from build123d import *

# Parameters (mm, degrees)
ESQUISSE1_R                                   = 3.9
BOSS_EXTRU_1_DEPTH                            = 105
ESQUISSE2_W                                   = 12
ESQUISSE2_H                                   = 12
BOSS_EXTRU_2_DEPTH                            = 5
ESQUISSE14_R                                  = 3.9
ESQUISSE14_R_2                                = 3
ENL_V_MAT_EXTRU_1_DEPTH                       = 6
CHANFREIN1_SIZE                               = 2
TROU_POUR_TARAUDAGE_POUR_TROU_TARAUD_M3_D     = 2.5
TROU_POUR_TARAUDAGE_POUR_TROU_TARAUD_M3_DEPTH = 12


with BuildPart() as part:
    # Esquisse1 → Boss.-Extru.1 (new body)
    with BuildSketch(Plane.XY):
        with Locations((-68.275651986, -15.580620135)):
            Circle(ESQUISSE1_R)
    extrude(amount=BOSS_EXTRU_1_DEPTH)

    # Esquisse2 → Boss.-Extru.2 (add)
    with BuildSketch(Plane.XY.offset(105)):
        with Locations((-68.275651986, -15.580620135)):
            Rectangle(ESQUISSE2_W, ESQUISSE2_H)
    extrude(amount=BOSS_EXTRU_2_DEPTH)

    # Esquisse14 → Enlèv. mat.-Extru.1 (cut)
    with BuildSketch(Plane(origin=(0, 0, 0), x_dir=(-1, 0, 0), z_dir=(0, 0, -1))):
        with Locations((68.275651986, -15.580620135)):
            Circle(ESQUISSE14_R)
        with Locations((68.275651986, -15.580620135)):
            Circle(ESQUISSE14_R_2, mode=Mode.SUBTRACT)
    extrude(amount=-ENL_V_MAT_EXTRU_1_DEPTH, mode=Mode.SUBTRACT)

    # Chanfrein1
    chanfrein1_edges = [part.edges().sort_by_distance(p)[0] for p in [
        (-62.275651986, -15.580620135, 110),
    ]]
    chamfer(chanfrein1_edges, length=CHANFREIN1_SIZE)

    # Trou pour taraudage pour trou taraudé M3x0.51
    with Locations(Plane(origin=(0, 0, 0), x_dir=(-1, 0, 0), z_dir=(0, 0, -1))):
        with Locations((68.275651986, -15.580620135)):
            Hole(TROU_POUR_TARAUDAGE_POUR_TROU_TARAUD_M3_D / 2, depth=TROU_POUR_TARAUDAGE_POUR_TROU_TARAUD_M3_DEPTH)


solid = part.part
Design review of the part built by this model. Coordinates are the model's own, in mm. A direction names the side the tool comes from. Round coordinates to 2 decimals unless told otherwise and drop trailing zeros. Write each loop counter-clockwise with the first axis right and the second up, starting at its lowest first coordinate (ties: lowest second). Pieces come first, ordered by that corner, then holes.
Item 1: For faces 5 (the flat face through (-68, -17, 0)), 6 (the flat face through (-71, -18, 6)), list the 3-axis set-ups (+Z, -Z, +X, -X, +Y, -Y) from which the entire face can be reached by the end or side of a thin tool; tool diameter is ignored.
Item 2: Consider section B-B on z = 83.5. Give the boundary of the cut face in (x, y).
Item 3: Draft analysis for pull direction Y (two halves, no side actions). For faces 1 (the flat face through (-68, -16, 12)), 2 (the cylindrical face through (-71.047, -16.73, 2.958)), 3 (the flat face through (-74.276, -16, 107)), 4 (the flat face through (-68, -21.581, 107)), state which applies: released by +Y, released by -Y, zero draft, split by the parting line, or undercut.
Item 4: Wall thickness on L1, parallel to Z at x = -64.5, y = -10.75; L2, parallel to X at y = -15.5, z = 104.5; L3, parallel to Z at x = -67.75, y = -14.75: over which ranges is each line inside the solid? List them lowest first.
Item 5: For pin 1 Ø1.5 at (y, z) = (-16, 28) entering from -X; pin 2 Ø1.5 at (x, y) = (-72.5, -14) entering from -Z; pin 3 Ø5 at (y, z) = (-16, 65.5) entering from +X, all flat-tipped, find the tip position at first contact; note any pin that passes through.
Item 6: Consider section A-A on z = 7. Give the boundary of the cut face in (x, y), and give its area (3 significant figures).
Check values:
1. face 5: -Z, +X, -X, +Y, -Y
1. face 6: -Z
2. outline: circle Ø7.8 at (-68.28, -15.58)
3. face 1: undercut
3. face 2: split by the parting line
3. face 3: zero draft
3. face 4: released by -Y
4. L1: z = 105 to 110
4. L2: x = -72.17 to -64.38
4. L3: z = 12 to 110
5. pin 1: stops at x = -72.18
5. pin 2: stops at z = 6
5. pin 3: stops at x = -64.38
6. outline: circle Ø7.8 at (-68.28, -15.58); hole circle Ø2.5 at (-68.28, -15.58)
6. area: 42.9 mm2
